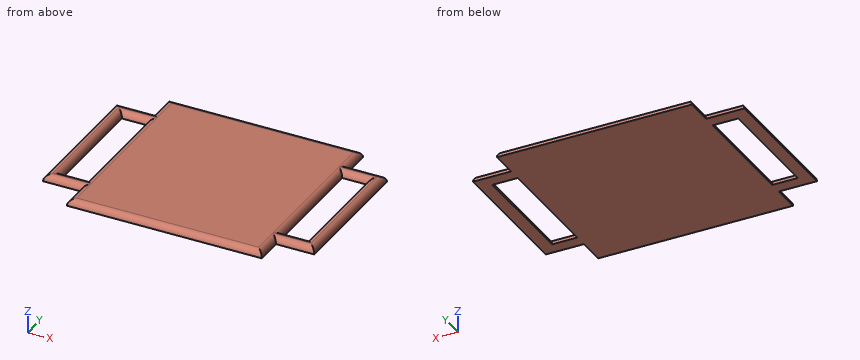
```python
from build123d import *

# Parameters (mm, degrees)
F2_DEPTH = 5
F3_R     = 4.99999


# Not quite as in the source:
# - a fillet or chamfer is up to 0.001 mm smaller than in the source, because OpenCascade refuses the exact size


with BuildPart() as f2:
    # F1 (on Top) → F2 (new body)
    with BuildSketch(Plane.XY):
        Polygon((-76.5, -76.5), (76.5, -76.5), (76.5, -55), (76.5, -45), (76.5, 45), (76.5, 55), (76.5, 76.5), (-76.5, 76.5), (-76.5, 55), (-76.5, 45), (-76.5, -45), (-76.5, -55), align=None)
        Polygon((76.5, -45), (76.5, -55), (106.5, -55), (106.5, 55), (76.5, 55), (76.5, 45), (96.5, 45), (96.5, -45), align=None)
        Polygon((-106.5, -55), (-76.5, -55), (-76.5, -45), (-96.5, -45), (-96.5, 45), (-76.5, 45), (-76.5, 55), (-106.5, 55), align=None)
    extrude(amount=F2_DEPTH)

    # F3 (radius 5 in the source; OpenCascade refuses exactly that, so slightly less here)
    f3_edges = [f2.edges().sort_by_distance(p)[0] for p in [
        (0, -76.5, 5),
        (76.5, -65.75, 5),
        (91.5, -55, 5),
        (106.5, 0, 5),
        (91.5, 55, 5),
        (76.5, 65.75, 5),
        (0, 76.5, 5),
        (-76.5, 65.75, 5),
        (-91.5, 55, 5),
        (-106.5, 0, 5),
        (-91.5, -55, 5),
        (-76.5, -65.75, 5),
        (-76.5, 0, 5),
        (-86.5, -45, 5),
        (-96.5, 0, 5),
        (-86.5, 45, 5),
        (76.5, 0, 5),
        (86.5, 45, 5),
        (96.5, 0, 5),
        (86.5, -45, 5),
    ]]
    fillet(f3_edges, radius=F3_R)


solid = f2.part
```
Design review of the part built by this model. Coordinates are the model's own, in mm. Give positions to 0.01 mm unless a question says otherwise; leave off trailing zeros. Loops run counter-clockwise (first coordinate to the right, second up) from the corner with the lowest first, then second, coordinate; pieces in that order, holes last. Notation, with made-up numbers: M 73.5,15.25 L 120.5,15.25 A30 cw 120.5,37.25 Z; hole C 24.5,33 d8. An arc over 180 degrees is marked long. Return JSON: item names as keys, results as strings. Group by question number.
Item 1: For probe 1 along X at (y, z) = (19.5, 0.9); probe 2 along X at (y, z) = (44, 3.15); probe 3 along Y at (x, z) = (-81, 2.1), list the stretches that pass through material, from the lowest coordinate up.
Item 2: We need section A-A (y = -42). Give the number of separate pieces and of enclosed holes in the cut face, and give its area (3 significant figures).
Item 3: We need section B-B (z = 2.65). Give the boundary of the cut face in (x, y).
Item 4: Insertion check: pin 1 Ø1 at (y, z) = (61, 3.5) entering from -X; pin 2 Ø2 at (x, z) = (37, 2) entering from -Y; pin 3 Ø8 at (x, y) = (-14.5, -50) entering from -Z; pin 4 Ø2 at (x, z) = (-28, 1.5) entering from -Y. Each pin has a flat end and moves straight along its axis. Give the tip position at first contact, or say it passes through.
Output:
{
 "1": {"probe 1": "x = -106.42 to -96.58, -76.42 to 76.42, 96.58 to 106.42", "probe 2": "x = -105.38 to -97.62, -75.38 to 75.38, 97.62 to 105.38", "probe 3": "y = -54.54 to -45.46, 45.46 to 54.54"},
 "2": {"separate pieces": "3", "enclosed holes": "0", "area": "833 mm^2"},
 "3": {"outline": "M -105.74,-54.24 L -75.74,-54.24 L -75.74,-75.74 L 75.74,-75.74 L 75.74,-54.24 L 105.74,-54.24 L 105.74,54.24 L 75.74,54.24 L 75.74,75.74 L -75.74,75.74 L -75.74,54.24 L -105.74,54.24 Z; hole M -97.26,-45.76 L -75.74,-45.76 L -75.74,45.76 L -97.26,45.76 Z; hole M 75.74,-45.76 L 97.26,-45.76 L 97.26,45.76 L 75.74,45.76 Z"},
 "4": {"pin 1": "stops at x = -75.5", "pin 2": "stops at y = -76.4", "pin 3": "stops at z = 0", "pin 4": "stops at y = -76.47"}
}
